Could you check a few things on this model? Use its own coordinates, in mm. Round coordinates to 2 decimals unless told otherwise and drop trailing zeros. Loops run counter-clockwise (first coordinate to the right, second up) from the corner with the lowest first, then second, coordinate; pieces in that order, holes last. Notation, with made-up numbers: (0, 63.25) -> (4, 63.25) arc R6 cw to (4, 74.25) -> close; hole circle Ø3 at (-7.75, 46). An arc over 180 degrees is marked (long way). One line per item, written item: value.
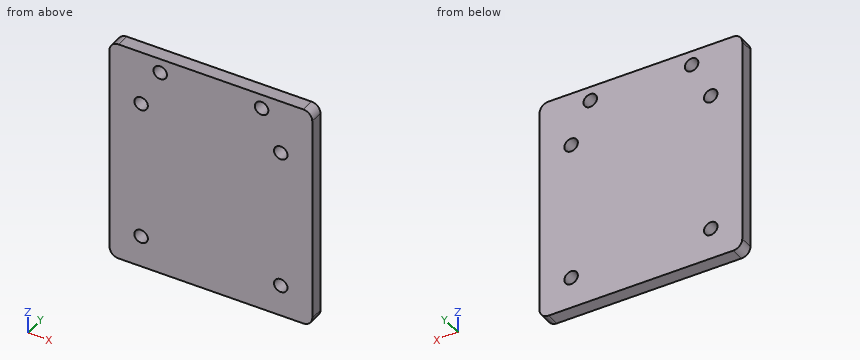
from build123d import *

# Parameters (mm, degrees)
SKETCH_W  = 45
SKETCH_H  = 50
SKETCH_R  = 1.5
PAD_DEPTH = 3
FILLET_R  = 2


with BuildPart() as part:
    # Sketch (on XZ_Plane of Origin) → Pad (new body)
    with BuildSketch(Plane.XZ):
        with Locations((0, 2.5)):
            Rectangle(SKETCH_W, SKETCH_H)
        with Locations((-15.5, 15.5)):
            Circle(SKETCH_R, mode=Mode.SUBTRACT)
        with Locations((15.5, 15.5)):
            Circle(SKETCH_R, mode=Mode.SUBTRACT)
        with Locations((15.5, -15.5)):
            Circle(SKETCH_R, mode=Mode.SUBTRACT)
        with Locations((-15.5, -15.5)):
            Circle(SKETCH_R, mode=Mode.SUBTRACT)
        with Locations((-11.25, 24.325)):
            Circle(SKETCH_R, mode=Mode.SUBTRACT)
        with Locations((11.25, 24.325)):
            Circle(SKETCH_R, mode=Mode.SUBTRACT)
    extrude(amount=PAD_DEPTH)

    # Fillet
    fillet_edges = [part.edges().sort_by_distance(p)[0] for p in [
        (22.5, -1.5, 27.5),
        (22.5, -1.5, -22.5),
        (-22.5, -1.5, -22.5),
        (-22.5, -1.5, 27.5),
    ]]
    fillet(fillet_edges, radius=FILLET_R)


solid = part.part
(1) I'm going to push a flat-ended pin straight in: pin 1 Ø2.5 at (x, z) = (15.5, -15.5) entering from +Y. Where does the tip first touch, or does it pass through?
Recorded:
pin 1: through
(2) If we section it at C-C, the plane y = -1.4: Please give me the cut outline in (x, z) (3 decimals).
Recorded:
outline: (-22.5, -20.5) arc R2 ccw to (-20.5, -22.5) -> (20.5, -22.5) arc R2 ccw to (22.5, -20.5) -> (22.5, 25.5) arc R2 ccw to (20.5, 27.5) -> (-20.5, 27.5) arc R2 ccw to (-22.5, 25.5) -> close; hole circle Ø3 at (-15.5, -15.5); hole circle Ø3 at (-15.5, 15.5); hole circle Ø3 at (-11.25, 24.325); hole circle Ø3 at (11.25, 24.325); hole circle Ø3 at (15.5, -15.5); hole circle Ø3 at (15.5, 15.5)
(3) If we section it at B-B, the plane z = -15.5: Please give me the cut outline in (x, y), then the cut area to 3 significant figures.
Recorded:
outline: (-22.5, -3) -> (-17, -3) -> (-17, 0) -> (-22.5, 0) -> close; (-14, -3) -> (14, -3) -> (14, 0) -> (-14, 0) -> close; (17, -3) -> (22.5, -3) -> (22.5, 0) -> (17, 0) -> close
area: 117 mm²
(4) If we section it at A-A, the plane x = 11.25: Please give me the cut outline in (y, z) (3 decimals).
Recorded:
outline: (-3, -22.5) -> (0, -22.5) -> (0, 22.825) -> (-3, 22.825) -> close; (-3, 25.825) -> (0, 25.825) -> (0, 27.5) -> (-3, 27.5) -> close
(5) If we section it at D-D, the plane z = 23.5: Please give me the cut outline in (x, y).
Recorded:
outline: (-22.5, -3) -> (-12.5, -3) -> (-12.5, 0) -> (-22.5, 0) -> close; (-10, -3) -> (10, -3) -> (10, 0) -> (-10, 0) -> close; (12.5, -3) -> (22.5, -3) -> (22.5, 0) -> (12.5, 0) -> close
(6) If I drill on L1, parallel to Z at x = -15.5, y = -0.7; L2, parallel to Z at x = 11.25, y = -2.3 (3 decimals); L3, parallel to Z at x = 15, y = -0.35, over which ranges is the centre line in solid material (lowest first)?
Recorded:
L1: -22.5 to -17, -14 to 14, 17 to 27.5
L2: -22.5 to 22.825, 25.825 to 27.5
L3: -22.5 to -16.91, -14.09 to 14.09, 16.91 to 27.5
